Verification items for the finished model (mm, model axes). Face numbers are marked on the shaded views. Give positions to 0.01 mm unless a question says otherwise; leave off trailing zeros. Write each loop counter-clockwise with the first axis right and the second up, starting at its lowest first coordinate (ties: lowest second). Pieces come first, ordered by that corner, then holes. Notation, with made-up numbers: (27.5, 81.5) -> (64.5, 81.5) arc R14 cw to (64.5, 87.5) -> close; hole circle Ø8 at (48, 35). An arc over 180 degrees is marked (long way). Answer as CSV lines item,"result".
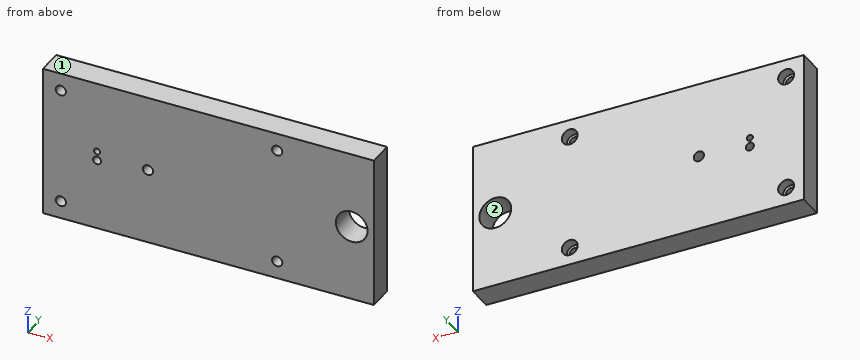
```python
from build123d import *

# Parameters (mm, degrees)
SKETCH1_W           = 165.1
SKETCH1_H           = 76.2
BOSS_EXTRUDE1_DEPTH = 12.7
SKETCH2_R           = 3.9624
SKETCH2_R_2         = 2.5527
CUT_EXTRUDE3_DEPTH  = 4.826
SKETCH10_R          = 2.5527
CUT_EXTRUDE9_DEPTH  = 22.352
SKETCH11_R          = 7.9375
SKETCH11_R_2        = 2.5527
SKETCH11_R_3        = 2.0193
SKETCH11_R_4        = 1.524
CUT_EXTRUDE10_DEPTH = 22.352


with BuildPart() as part:
    # Sketch1 → Boss-Extrude1 (new body)
    with BuildSketch(Plane(origin=(0, 0, 0), x_dir=(1, 0, 0), z_dir=(0, 1, 0))):
        with Locations((17.306400742, -14.73812616)):
            Rectangle(SKETCH1_W, SKETCH1_H)
    extrude(amount=BOSS_EXTRUDE1_DEPTH)

    # Sketch2 → Cut-Extrude3 (cut)
    # profile 1 of 4: a face of its own
    with BuildSketch(Plane(origin=(0, 12.7, 0), x_dir=(1, 0, 0), z_dir=(0, 1, 0))):
        with Locations(Location((-56.353599258, -43.94812616, 0), (0, 0, 270))):
            Circle(SKETCH2_R)
        with Locations(Location((-56.353599258, -43.94812616, 0), (0, 0, 270))):
            Circle(SKETCH2_R_2, mode=Mode.SUBTRACT)
    # profile 2 of 4: a face of its own
    with BuildSketch(Plane(origin=(0, 12.7, 0), x_dir=(1, 0, 0), z_dir=(0, 1, 0))):
        with Locations(Location((-56.353599258, 14.47187384, 0), (0, 0, 270))):
            Circle(SKETCH2_R)
        with Locations(Location((-56.353599258, 14.47187384, 0), (0, 0, 270))):
            Circle(SKETCH2_R_2, mode=Mode.SUBTRACT)
    # profile 3 of 4: a face of its own
    with BuildSketch(Plane(origin=(0, 12.7, 0), x_dir=(1, 0, 0), z_dir=(0, 1, 0))):
        with Locations(Location((51.596400742, 14.47187384, 0), (0, 0, 270))):
            Circle(SKETCH2_R)
        with Locations(Location((51.596400742, 14.47187384, 0), (0, 0, 270))):
            Circle(SKETCH2_R_2, mode=Mode.SUBTRACT)
    # profile 4 of 4: a face of its own
    with BuildSketch(Plane(origin=(0, 12.7, 0), x_dir=(1, 0, 0), z_dir=(0, 1, 0))):
        with Locations(Location((51.596400742, -43.94812616, 0), (0, 0, 270))):
            Circle(SKETCH2_R)
        with Locations(Location((51.596400742, -43.94812616, 0), (0, 0, 270))):
            Circle(SKETCH2_R_2, mode=Mode.SUBTRACT)
    extrude(amount=-CUT_EXTRUDE3_DEPTH, mode=Mode.SUBTRACT)

    # Sketch10 → Cut-Extrude9 (cut)
    with BuildSketch(Plane(origin=(0, 12.7, 0), x_dir=(1, 0, 0), z_dir=(0, 1, 0))):
        with Locations(Location((-56.353599258, -43.94812616, 0), (0, 0, 270))):
            Circle(SKETCH10_R)
        with Locations(Location((-56.353599258, 14.47187384, 0), (0, 0, 270))):
            Circle(SKETCH10_R)
        with Locations(Location((51.596400742, 14.47187384, 0), (0, 0, 270))):
            Circle(SKETCH10_R)
        with Locations(Location((51.596400742, -43.94812616, 0), (0, 0, 270))):
            Circle(SKETCH10_R)
    extrude(amount=-CUT_EXTRUDE9_DEPTH, mode=Mode.SUBTRACT)

    # Sketch11 → Cut-Extrude10 (cut)
    with BuildSketch(Plane(origin=(0, 12.7, 0), x_dir=(1, 0, 0), z_dir=(0, 1, 0))):
        with Locations(Location((88.743900742, -14.73812616, 0), (0, 0, 270))):
            Circle(SKETCH11_R)
        with Locations(Location((-12.856099258, -14.73812616, 0), (0, 0, 270))):
            Circle(SKETCH11_R_2)
        with Locations(Location((-38.256099258, -12.40132616, 0), (0, 0, 270))):
            Circle(SKETCH11_R_3)
        with Locations(Location((-38.256099258, -17.07492616, 0), (0, 0, 270))):
            Circle(SKETCH11_R_4)
    extrude(amount=-CUT_EXTRUDE10_DEPTH, mode=Mode.SUBTRACT)


solid = part.part
```
1) Depth check by flat-ended pin: pin 1 (6 mm diameter, centred on x = -56.35, z = 43.95, fed in from +Y); pin 2 (5 mm diameter, centred on x = 51.6, z = -14.47, fed in from +Y). Enter the tip coordinate at first touch or a pass-through.
Reported:
pin 1,"y = 7.87"
pin 2,"through"
2) Draft check along X on the marked faces 1 and 2. Enter one of: +X half, -X half, draft (parallel to the pull), parting line (faces both ways), or undercut.
Reported:
face 1,"draft"
face 2,"undercut"
3) Section check A-A (z = 21). Record the boundary of the cut face in (x, y).
Reported:
outline,"(-65.24, 0) -> (83.87, 0) -> (83.87, 12.7) -> (-65.24, 12.7) -> close; (93.62, 0) -> (99.86, 0) -> (99.86, 12.7) -> (93.62, 12.7) -> close"
4) Section check B-B (x = 87). Record the boundary of the cut face in (y, z), and give its area (3 significant figures).
Reported:
outline,"(0, -23.36) -> (12.7, -23.36) -> (12.7, 6.99) -> (0, 6.99) -> close; (0, 22.48) -> (12.7, 22.48) -> (12.7, 52.84) -> (0, 52.84) -> close"
area,"771 mm²"
5) Section check C-C (y = 3.75). State how many separate pieces and enclosed holes the cut face has, and give its area (3 significant figures).
Reported:
separate pieces,"1"
enclosed holes,"8"
area,"12,300 mm²"
6) Scan lines: line 1 along Z through (x, y) = (-38, 7.5); line 2 along Z through (x, y) = (-58.5, 10.5); line 3 along X through (y, z) = (7.75, -15.5). Record each from-to range of solid material in increasing order.
Reported:
line 1,"-23.36 to 10.4, 14.4 to 15.57, 18.58 to 52.84"
line 2,"-23.36 to -17.8, -11.14 to 40.62, 47.28 to 52.84"
line 3,"-65.24 to -58.69, -54.02 to 49.26, 53.93 to 99.86"
